```python
from build123d import *

# Parameters (mm, degrees)
SWEEP1_START       = -204.68052275
SWEEP1_OUTLINE_R   = 13.5
SWEEP1_OUTLINE_R_2 = 2.5
SWEEP1_DEPTH       = 204.68052275


# Read off the part's stored shape, not the designer's step: Sweep1
with BuildPart() as part:
    # Sketch1 → Revolve1 (revolve)
    with BuildSketch(Plane.XY, mode=Mode.PRIVATE) as revolve1_sk:
        with BuildLine():
            Line((-13, 98.3), (-18.085, 98.3))
            Line((-18.085, 98.3), (-19.1, 73.3))
            Line((-19.1, 73.3), (-31.5, 73.3))
            Line((-31.5, 73.3), (-31.5, 58.3))
            Line((-31.5, 58.3), (-27.5, 56.8))
            Line((-27.5, 56.8), (-27.5, 52.8))
            Line((-27.5, 52.8), (-31.5, 51.3))
            Line((-31.5, 51.3), (-31.5, 46.3))
            Line((-31.5, 46.3), (-25, 46.3))
            Line((-25, 46.3), (-25, 35.3))
            Line((-25, 35.3), (-20, 30.3))
            Line((-20, 30.3), (-20, 22.3))
            Line((-20, 22.3), (-24.75, 22.3))
            ThreePointArc((-24.75, 22.3), (-24.926776695, 22.226776695), (-25, 22.05))
            Line((-25, 22.05), (-25, 2.444337567))
            ThreePointArc((-25, 2.444337567), (-24.966506351, 2.319337567), (-24.875, 2.227831216))
            Line((-24.875, 2.227831216), (-20.669872981, -0.2))
            Line((-20.669872981, -0.2), (-13.5, -0.2))
            Line((-13.5, -0.2), (-13.5, 0))
            Line((-13.5, 0), (-2.5, 0))
            Line((-2.5, 0), (-2.5, 15))
            Line((-2.5, 15), (0, 15))
            Line((0, 15), (0, 64.3))
            Line((0, 64.3), (-13, 64.3))
            Line((-13, 64.3), (-13, 69.3))
            Line((-13, 69.3), (-14, 69.3))
            ThreePointArc((-14, 69.3), (-15.414213562, 69.885786438), (-16, 71.3))
            Line((-16, 71.3), (-16, 89.3))
            ThreePointArc((-16, 89.3), (-15.414213562, 90.714213562), (-14, 91.3))
            Line((-14, 91.3), (-13, 91.3))
            Line((-13, 91.3), (-13, 98.3))
        make_face()
    revolve(revolve1_sk.sketch.rotate(Axis((0, 0, 0), (0, 1, 0)), 270), axis=Axis((0, 0, 0), (0, 1, 0)))

    # Sweep1 outline → Sweep1 (add)
    with BuildSketch(Plane(origin=(0, 0, 0), x_dir=(1, 0, 0), z_dir=(0, 1, 0)).offset(SWEEP1_START)):
        Circle(SWEEP1_OUTLINE_R)
        Circle(SWEEP1_OUTLINE_R_2, mode=Mode.SUBTRACT)
    extrude(amount=SWEEP1_DEPTH)


solid = part.part
```
Design review of the part built by this model. Coordinates are the model's own, in mm. A direction names the side the tool comes from. Coordinates: 2 decimals unless noted, no trailing zeros. Order: outer loops, then holes, each group sorted by start corner. A loop starts at its lowest first (then second) coordinate and runs counter-clockwise, first axis right, second up. Notation, with made-up numbers: (62.5, 1.25) - (90.5, 1.25) arc R22 ccw to (90.5, 34.25) - close; hole circle Ø3 at (-20.75, 8.5). An arc over 180 degrees is marked (long way). Answer in a Markdown table with one row per item.
(1) The part is to be moulded in two halves that separate along Y. For faces 1 (the cylindrical face through (-7.509, 40.723, -23.846)), 2 (the flat face through (3, -204.681, 0)), 3 (the conical face through (-6.08, 30.543, -19.308)), 4 (the flat face through (9.3, 91.3, -9.3)), say which applies: released by +Y, released by -Y, zero draft, split by the parting line, or undercut.
Checked values:
| item | result |
|---|---|
| face 1 | zero draft |
| face 2 | released by -Y |
| face 3 | undercut |
| face 4 | undercut |
(2) Wall thickness on line 1 along X through (y, z) = (-128, 0); line 2 along Z through (x, y) = (0.5, -188); line 3 along Y through (x, z) = (7, 11): over which ranges is each line inside the solid? List them lowest first. Write a range as from..to.
Checked values:
| item | result |
|---|---|
| line 1 | -13.5..-2.5, 2.5..13.5 |
| line 2 | -13.49..-2.45, 2.45..13.49 |
| line 3 | -204.68..69.3, 91.3..98.3 |
(3) Clearance check with flat-ended pins moving along their axes: pin 1 (10 mm diameter, centred on y = 67.5, z = -11.5, fed in from +X); pin 2 (8 mm diameter, centred on x = -5, z = -5, fed in from +Y); pin 3 (2 mm diameter, centred on x = -15, y = -8.5, fed in from +Z); pin 4 (5 mm diameter, centred on x = 3.5, y = -106, fed in from -Z). State where each tip first meets the part, or that it passes through.
Checked values:
| item | result |
|---|---|
| pin 1 | x = 30.82 |
| pin 2 | y = 64.3 |
| pin 3 | through |
| pin 4 | z = -13.46 |
(4) For faces 5 (the cylindrical face through (7.91, 94.849, 10.316)), 6 (the cylindrical face through (15.62, 80.43, 3.47)), 7 (the cylindrical face through (-7.509, 12.11, -23.846)), list the 3-axis set-ups (+Z, -Z, +X, -X, +Y, -Y) from which the entire face can be reached by the end or side of a thin tool; tool diameter is ignored.
Checked values:
| item | result |
|---|---|
| face 5 | +Y |
| face 6 | none |
| face 7 | -Y |
(5) Consider section A-A on y = -145. State the section outline as (x, z) points, plus the area to 3 significant figures.
Checked values:
| item | result |
|---|---|
| outline | circle Ø27 at (0, 0); hole circle Ø5 at (0, 0) |
| area | 553 mm^2 |
